from build123d import *

# Parameters (mm, degrees)
SKETCH_1_R      = 6.5
SKETCH_1_R_2    = 3
EXTRUDE_1_DEPTH = 5
CHAMFER_1_SIZE  = 0.2


with BuildPart() as part:
    # 草图1 → 凸台-拉伸1 (new body)
    with BuildSketch(Plane(origin=(0, 0, 0), x_dir=(1, 0, 0), z_dir=(0, 1, 0))):
        with Locations(Location((0, 0, 0), (0, 0, 270))):
            Circle(SKETCH_1_R)
        with Locations(Location((0, 0, 0), (0, 0, 270))):
            Circle(SKETCH_1_R_2, mode=Mode.SUBTRACT)
    extrude(amount=EXTRUDE_1_DEPTH)

    # 草图2 → 切除-旋转1 (revolve, cut)
    with BuildSketch(Plane(origin=(0, 0, 0), x_dir=(0, 0, -1), z_dir=(1, 0, 0)), mode=Mode.PRIVATE) as cut_revolve_1_sk:
        Polygon((-5.717819926, 5), (-5.55, 4.8), (-3.95, 4.8), (-3.782180074, 5), align=None)
        Polygon((-3.95, 0.2), (-3.782180074, 0), (-5.717819926, 0), (-5.55, 0.2), align=None)
    revolve(cut_revolve_1_sk.sketch.rotate(Axis((0, 0, 0), (0, 1, 0)), 180), axis=Axis((0, 0, 0), (0, 1, 0)), mode=Mode.SUBTRACT)

    # 倒角1
    chamfer_1_edges = [part.edges().sort_by_distance(p)[0] for p in [
        (0, 0, -6.5),
        (0, 5, -6.5),
    ]]
    chamfer(chamfer_1_edges, length=CHAMFER_1_SIZE)


solid = part.part
Read the model definition and answer for the solid it produces. Units are mm, in the model's axes. Coordinates: 2 decimals unless noted, no trailing zeros. Order: outer loops, then holes, each group sorted by start corner. A loop starts at its lowest first (then second) coordinate and runs counter-clockwise, first axis right, second up. Notation, with made-up numbers: (-22.5, 82.5) -> (31.5, 82.5) arc R9 cw to (31.5, 89.5) -> close; hole circle Ø6 at (-4.5, 48). An arc over 180 degrees is marked (long way). Answer as a JSON object with one key per item and string values.
1) A cutting plane is placed at C-C, the plane y = 3.4. Determine the outline of the cut face in (x, z), plus the area to 3 significant figures.
Model answer:
{"outline": "circle Ø13 at (0, 0); hole circle Ø6 at (0, 0)", "area": "104 mm²"}
2) Consider line 1 along X through (y, z) = (1.8, 0); line 2 along Y through (x, z) = (1.75, 4); line 3 along Z through (x, y) = (-0.5, 2.5). Determine where each line is inside the solid, lowest interval first. Write a range as from..to.
Model answer:
{"line 1": "x = -6.5..-3, 3..6.5", "line 2": "y = 0.2..4.8", "line 3": "z = -6.48..-2.96, 2.96..6.48"}
3) A cutting plane is placed at B-B, the plane z = 0. Determine the outline of the cut face in (x, y), plus the area to 3 significant figures.
Model answer:
{"outline": "(-6.5, 0.2) -> (-6.3, 0) -> (-5.72, 0) -> (-5.55, 0.2) -> (-3.95, 0.2) -> (-3.78, 0) -> (-3, 0) -> (-3, 5) -> (-3.78, 5) -> (-3.95, 4.8) -> (-5.55, 4.8) -> (-5.72, 5) -> (-6.3, 5) -> (-6.5, 4.8) -> close; (3, 0) -> (3.78, 0) -> (3.95, 0.2) -> (5.55, 0.2) -> (5.72, 0) -> (6.3, 0) -> (6.5, 0.2) -> (6.5, 4.8) -> (6.3, 5) -> (5.72, 5) -> (5.55, 4.8) -> (3.95, 4.8) -> (3.78, 5) -> (3, 5) -> close", "area": "33.5 mm²"}
4) Each of these flat-tipped pins is pushed along its axis until it touches: pin 1 (1 mm diameter, centred on x = 2.5, y = 2.5, fed in from -Z); pin 2 (1 mm diameter, centred on x = 5, y = 3.5, fed in from -Z); pin 3 (1 mm diameter, centred on x = 3.5, y = 2.5, fed in from -Z). Where does it stop, or does it pass through?
Model answer:
{"pin 1": "stops at z = -6.18", "pin 2": "stops at z = -4.69", "pin 3": "stops at z = -5.77"}
5) A cutting plane is placed at A-A, the plane x = 0. Determine the outline of the cut face in (y, z).
Model answer:
{"outline": "(0, -6.3) -> (0.2, -6.5) -> (4.8, -6.5) -> (5, -6.3) -> (5, -5.72) -> (4.8, -5.55) -> (4.8, -3.95) -> (5, -3.78) -> (5, -3) -> (0, -3) -> (0, -3.78) -> (0.2, -3.95) -> (0.2, -5.55) -> (0, -5.72) -> close; (0, 3) -> (5, 3) -> (5, 3.78) -> (4.8, 3.95) -> (4.8, 5.55) -> (5, 5.72) -> (5, 6.3) -> (4.8, 6.5) -> (0.2, 6.5) -> (0, 6.3) -> (0, 5.72) -> (0.2, 5.55) -> (0.2, 3.95) -> (0, 3.78) -> close"}
6) The mould has two halves that part along Z. Classify faces 1 (the face through (-4, 0.2, -1)), 2 (the face through (-3.955, 2.468, -5.158)), 3 (the face through (3, 0, -1)), 4 (the face through (-4, 4.8, -1)): released by +Z, released by -Z, zero draft, split by the parting line, or undercut.
Model answer:
{"face 1": "undercut", "face 2": "split by the parting line", "face 3": "zero draft", "face 4": "undercut"}
